Part model, mm, in its own coordinate system. Coordinates: 2 decimals unless noted, no trailing zeros. Loops run counter-clockwise (first coordinate to the right, second up) from the corner with the lowest first, then second, coordinate; pieces in that order, holes last. Notation, with made-up numbers: (81.25, 79.5) - (90.25, 79.5) arc R16 cw to (90.25, 107.5) - close; hole circle Ø4 at (63.25, 15). An arc over 180 degrees is marked (long way). Use a Markdown table: item, result. Add a question column.
1. Band-saw the part on A-A, the plane z = 18.25. Give the cut face in (x, y), plus the area to 3 significant figures.
2. Band-saw the part on B-B, the plane x = 3.25. Count the separate pieces of the cut face and the enclosed holes in it, plus the area to 4 significant figures.
3. Band-saw the part on C-C, the plane z = 0. Give the cut face in (x, y).
4. Pull direction Y, two halves, no side cores. Call faces 1 (the cylindrical face through (3, 25, 54)), 2 (the cylindrical face through (3.13, -1.4, -40.17)), 3 (the flat face through (3, 0, -55)): pulls with the +Y half, pulls with the -Y half, needs draft (parallel to the pull), parting line crosses it, or undercut.
5. Wall check: probe 1 along Y at (x, z) = (2, -22); probe 2 along Y at (x, z) = (3, 18.25); probe 3 along Z at (x, y) = (3.5, 13.5). Give the ranges that are in metal, low to high. Write a range as [from, to].
from build123d import *

# Parameters (mm, degrees)
SKETCH1_W              = 110
SKETCH1_H              = 54
BOSS_EXTRUDE1_DEPTH    = 6.35
FILLET1_R              = 5
F_6_CLEARANCE_HOLE1_D  = 3.6576
SKETCH5_R              = 5
CUT_EXTRUDE1_DEPTH     = 7.35
F_6_CLEARANCE_HOLE2_D  = 3.6576
F_10_CLEARANCE_HOLE1_D = 4.9784


with BuildPart() as part:
    # Sketch1 → Boss-Extrude1 (new body)
    with BuildSketch(Plane(origin=(0, 0, 0), x_dir=(0, 0, -1), z_dir=(1, 0, 0))):
        Rectangle(SKETCH1_W, SKETCH1_H)
    extrude(amount=BOSS_EXTRUDE1_DEPTH)

    # Fillet1
    fillet1_edges = [part.edges().sort_by_distance(p)[0] for p in [
        (3.175, -27, -55),
        (3.175, -27, 55),
        (3.175, 27, 55),
        (3.175, 27, -55),
    ]]
    fillet(fillet1_edges, radius=FILLET1_R)

    # #6 Clearance Hole1 (through all)
    with Locations(Plane(origin=(6.35, 0, 0), x_dir=(0, 0, -1), z_dir=(1, 0, 0))):
        with Locations((-22, 22), (22, 22), (22, -22), (-22, -22)):
            Hole(F_6_CLEARANCE_HOLE1_D / 2)

    # Sketch5 → Cut-Extrude1 (cut, through all)
    with BuildSketch(Plane(origin=(6.35, 0, 0), x_dir=(0, 0, -1), z_dir=(1, 0, 0))):
        Circle(SKETCH5_R)
    extrude(amount=-CUT_EXTRUDE1_DEPTH, mode=Mode.SUBTRACT)

    # #6 Clearance Hole2 (through all)
    with Locations(Plane(origin=(6.35, 0, 0), x_dir=(0, 0, -1), z_dir=(1, 0, 0))):
        with Locations((-41.914797213, 11.884797213), (-28.085202787, 11.884797213), (-28.085202787, -1.944797213), (-41.914797213, -1.944797213), (28.085202787, 11.884797213), (28.085202787, -1.944797213), (41.914797213, -1.944797213), (41.914797213, 11.884797213)):
            Hole(F_6_CLEARANCE_HOLE2_D / 2)

    # #10 Clearance Hole1 (through all)
    with Locations(Plane.ZY):
        with Locations((18.25, 0), (-18.25, 0)):
            Hole(F_10_CLEARANCE_HOLE1_D / 2)


solid = part.part
Geometry check:
| question | item | result |
|---|---|---|
| 1 | outline | (0, -27) - (6.35, -27) - (6.35, -2.49) - (0, -2.49) - close; (0, 2.49) - (6.35, 2.49) - (6.35, 27) - (0, 27) - close |
| 1 | area | 311 mm^2 |
| 2 | separate pieces | 1 |
| 2 | enclosed holes | 15 |
| 2 | area | 5,675 mm^2 |
| 3 | outline | (0, -27) - (6.35, -27) - (6.35, -5) - (0, -5) - close; (0, 5) - (6.35, 5) - (6.35, 27) - (0, 27) - close |
| 4 | face 1 | pulls with the +Y half |
| 4 | face 2 | undercut |
| 4 | face 3 | needs draft |
| 5 | probe 1 | y = [-27, -23.83], [-20.17, 20.17], [23.83, 27] |
| 5 | probe 2 | y = [-27, -2.49], [2.49, 27] |
| 5 | probe 3 | z = [-55, -42.77], [-41.06, -28.94], [-27.23, 27.23], [28.94, 41.06], [42.77, 55] |
